```python
from build123d import *

# Parameters (mm, degrees)
CYLINDER074_R          = 1.75
CYLINDER074_DEPTH      = 30
CYLINDER074_ROLL_ANGLE = 90
CYLINDER073_R          = 1.75
CYLINDER073_DEPTH      = 30
CYLINDER073_ROLL_ANGLE = 90
BOX067_W               = 7.5
BOX067_H               = 2
BOX067_DEPTH           = 19
CHAMFER012_SIZE        = 2.5


with BuildPart() as cylinder186:
    # Cylinder074 → Cylinder074 (new body)
    with BuildSketch(Plane.XY):
        Circle(CYLINDER074_R)
    extrude(amount=CYLINDER074_DEPTH)


with BuildPart() as cylinder186_1:
    # Cylinder074 roll: moved
    add(cylinder186.part.rotate(Axis((0, 0, 0), (1, 0, 0)), CYLINDER074_ROLL_ANGLE))


with BuildPart() as cylinder186_2:
    # Cylinder074 placement: moved
    add(cylinder186_1.part.moved(Location((17.5, -21, -22.5))))


with BuildPart() as fusion060:
    # Cylinder073 → Cylinder073 (new body)
    with BuildSketch(Plane.XY):
        Circle(CYLINDER073_R)
    extrude(amount=CYLINDER073_DEPTH)


with BuildPart() as fusion060_1:
    # Cylinder073 roll: moved
    add(fusion060.part.rotate(Axis((0, 0, 0), (1, 0, 0)), CYLINDER073_ROLL_ANGLE))


with BuildPart() as fusion060_2:
    # Cylinder073 placement: moved
    add(fusion060_1.part.moved(Location((17.5, -21, -12.5))))

    # Fusion060: union Cylinder186
    add(cylinder186_2.part)


with BuildPart() as spacer:
    # Box067 → Box067 (new body)
    with BuildSketch(Plane(origin=(13.5, -39, -27), x_dir=(1, 0, 0), z_dir=(0, 0, 1))):
        with Locations((3.75, 1)):
            Rectangle(BOX067_W, BOX067_H)
    extrude(amount=BOX067_DEPTH)

    # Chamfer012
    chamfer012_edges = [spacer.edges().sort_by_distance(p)[0] for p in [
        (21, -38, -8),
        (21, -38, -27),
    ]]
    chamfer(chamfer012_edges, length=CHAMFER012_SIZE)

    # Cut094: cut Fusion060
    add(fusion060_2.part, mode=Mode.SUBTRACT)


solid = spacer.part
```
Design review of the part built by this model. Coordinates are the model's own, in mm. Coordinates: 2 decimals unless noted, no trailing zeros. Loops run counter-clockwise (first coordinate to the right, second up) from the corner with the lowest first, then second, coordinate; pieces in that order, holes last.
Q1. We need section C-C on x = 17.5. State the section outline as (y, z) points, and give its area (3 significant figures).
Reported:
outline: (-39, -27) - (-37, -27) - (-37, -24.25) - (-39, -24.25) - close; (-39, -20.75) - (-37, -20.75) - (-37, -14.25) - (-39, -14.25) - close; (-39, -10.75) - (-37, -10.75) - (-37, -8) - (-39, -8) - close
area: 24.0 mm2
Q2. We need section A-A on z = -22.5. State the section outline as (x, y) points, and give its area (3 significant figures).
Reported:
outline: (13.5, -39) - (15.75, -39) - (15.75, -37) - (13.5, -37) - close; (19.25, -39) - (21, -39) - (21, -37) - (19.25, -37) - close
area: 8.00 mm2
Q3. We need section D-D on x = 18.75. State the section outline as (y, z) points.
Reported:
outline: (-39, -26.75) - (-37, -26.75) - (-37, -23.72) - (-39, -23.72) - close; (-39, -21.28) - (-37, -21.28) - (-37, -13.72) - (-39, -13.72) - close; (-39, -11.28) - (-37, -11.28) - (-37, -8.25) - (-39, -8.25) - close
Q4. The part is to be moulded in two halves that separate along X. For faces 1 (the face through (16.21, -37.99, -11.32)), 2 (the face through (19.7, -38, -9.2)), 3 (the face through (17.272, -37.986, -20.765)), 4 (the face through (16, -38, -27)), say which applies: +X half, -X half, draft (parallel to the pull), parting line (faces both ways), or undercut.
Reported:
face 1: undercut
face 2: +X half
face 3: undercut
face 4: draft
Q5. To check wall thickness, follow line 1 (Z direction, x = 17.5, y = -38.5); line 2 (X direction, y = -38.25, z = -22.5); line 3 (Z direction, x = 16.5, y = -38.6). State the ranges of each line that lie inside material, in increasing order.
Reported:
line 1: z = -27 to -24.25, -20.75 to -14.25, -10.75 to -8
line 2: x = 13.5 to 15.75, 19.25 to 21
line 3: z = -27 to -23.94, -21.06 to -13.94, -11.06 to -8
Q6. We need section B-B on y = -38.2. State the section outline as (x, z) points.
Reported:
outline: (13.5, -27) - (18.5, -27) - (21, -24.5) - (21, -10.5) - (18.5, -8) - (13.5, -8) - close; hole circle Ø3.5 at (17.5, -22.5); hole circle Ø3.5 at (17.5, -12.5)
